Here's how the part is built. I have some questions about the finished solid (model axes, mm). A direction names the side the tool comes from. Round coordinates to 2 decimals unless told otherwise and drop trailing zeros. Loops run counter-clockwise (first coordinate to the right, second up) from the corner with the lowest first, then second, coordinate; pieces in that order, holes last. Notation, with made-up numbers: M 25.5,66.25 L 70.5,66.25 A16 ccw 70.5,90.25 Z; hole C 25,-34.5 d7. An arc over 180 degrees is marked long. Write each question's results on one line, items separated by ' | '. Start each with the question number.
```python
from build123d import *

# Parameters (mm, degrees)
SKETCH_1_W          = 20
SKETCH_1_H          = 10
SKETCH_1_W_2        = 18
SKETCH_1_H_2        = 8
EXTRUDE_1_DEPTH     = 80
SKETCH_3_R          = 1.6
SKETCH_3_R_2        = 2.6
CUT_EXTRUDE_1_DEPTH = 84.066238629


with BuildPart() as part:
    # 草图1 → 拉伸-薄壁1 (new body)
    with BuildSketch(Plane.XY):
        with Locations((10, -5)):
            Rectangle(SKETCH_1_W, SKETCH_1_H)
        with Locations((10, -5)):
            Rectangle(SKETCH_1_W_2, SKETCH_1_H_2, mode=Mode.SUBTRACT)
    extrude(amount=EXTRUDE_1_DEPTH)

    # 草图3 → 切除-拉伸1 (cut, through all)
    with BuildSketch(Plane(origin=(0, 0, 0), x_dir=(1, 0, 0), z_dir=(0, 1, 0))):
        with Locations(Location((5, -5, 0), (0, 0, 270))):
            Circle(SKETCH_3_R)
        with Locations(Location((15, -5, 0), (0, 0, 90))):
            Circle(SKETCH_3_R)
        with Locations(Location((15, -15, 0), (0, 0, 270))):
            Circle(SKETCH_3_R)
        with Locations(Location((5, -15, 0), (0, 0, 90))):
            Circle(SKETCH_3_R)
        with Locations(Location((10, -69, 0), (0, 0, 270))):
            Circle(SKETCH_3_R_2)
        with Locations(Location((10, -39, 0), (0, 0, 270))):
            Circle(SKETCH_3_R_2)
    extrude(amount=-CUT_EXTRUDE_1_DEPTH, mode=Mode.SUBTRACT)


solid = part.part
```
Item 1: I'm going to push a flat-ended pin straight in: pin 1 (1.9 mm diameter, centred on x = 5, z = 5, fed in from -Y). Where does the tip first touch, or does it pass through?
Item 2: If we section it at B-B on y = -3: Please give me the cut outline in (x, z).
Item 3: If we mould it in two halves opening along Y, with no side actions, what happens to faces 1 (the face through (1, -5, 39)), 2 (the face through (20, -5, 39)), 3 (the face through (14, 0, 39))? For each: released by +Y, released by -Y, zero draft, split by the parting line, or undercut.
Item 4: If we section it at A-A on x = 10: Please give me the cut outline in (y, z).
Item 5: If we section it at C-C on z = 63.5: Please give me the cut outline in (x, y).
Item 6: If we section it at D-D on z = 15: Please give me the cut outline in (x, y), and give its area (3 significant figures).
Item 7: I need wall thicknesses on L1, parallel to X at y = -0.5, z = 5; L2, parallel to Y at x = 16, z = 57; L3, parallel to X at y = -6, z = 38.5. Which ranges of each line are inside material? Lowest first, please.
Item 8: Which directions (+Z, -Z, +X, -X, +Y, -Y) give clear straight access to the entire face, cutting with the end or side of a thin tool? Please do faces 4 (the face through (10, -9.4, 80)), 5 (the face through (14, -9, 39)).
Numbers:
1) pin 1: through
2) outline: M 0,0 L 1,0 L 1,80 L 0,80 Z; M 19,0 L 20,0 L 20,80 L 19,80 Z
3) face 1: undercut | face 2: zero draft | face 3: released by +Y
4) outline: M -10,0 L -9,0 L -9,36.4 L -10,36.4 Z; M -10,41.6 L -9,41.6 L -9,66.4 L -10,66.4 Z; M -10,71.6 L -9,71.6 L -9,80 L -10,80 Z; M -1,0 L 0,0 L 0,36.4 L -1,36.4 Z; M -1,41.6 L 0,41.6 L 0,66.4 L -1,66.4 Z; M -1,71.6 L 0,71.6 L 0,80 L -1,80 Z
5) outline: M 0,-10 L 20,-10 L 20,0 L 0,0 Z; hole M 1,-9 L 19,-9 L 19,-1 L 1,-1 Z
6) outline: M 0,-10 L 3.4,-10 L 3.4,-9 L 1,-9 L 1,-1 L 3.4,-1 L 3.4,0 L 0,0 Z; M 6.6,-10 L 13.4,-10 L 13.4,-9 L 6.6,-9 Z; M 6.6,-1 L 13.4,-1 L 13.4,0 L 6.6,0 Z; M 16.6,-10 L 20,-10 L 20,0 L 16.6,0 L 16.6,-1 L 19,-1 L 19,-9 L 16.6,-9 Z | area: 43.2 mm²
7) L1: 0 to 3.4, 6.6 to 13.4, 16.6 to 20 | L2: -10 to -9, -1 to 0 | L3: 0 to 1, 19 to 20
8) face 4: +Z, +X, -X, +Y, -Y | face 5: +Z, -Z
